from build123d import *

# Parameters (mm, degrees)
SKETCH_1_R      = 150
SKETCH_1_R_2    = 3
SKETCH_1_R_3    = 1.55
SKETCH_1_R_4    = 1
EXTRUDE_1_DEPTH = 3


with BuildPart() as part:
    # 草图1 → 凸台-拉伸1 (new body)
    with BuildSketch(Plane(origin=(0, 0, 0), x_dir=(1, 0, 0), z_dir=(0, 1, 0))):
        with Locations(Location((0, 0, 0), (0, 0, 270))):
            Circle(SKETCH_1_R)
        with Locations(Location((0, 0, 0), (0, 0, 270))):
            Circle(SKETCH_1_R_2, mode=Mode.SUBTRACT)
        with Locations(Location((0, 10, 0), (0, 0, 270))):
            Circle(SKETCH_1_R_3, mode=Mode.SUBTRACT)
        with Locations(Location((10, 0, 0), (0, 0, 270))):
            Circle(SKETCH_1_R_3, mode=Mode.SUBTRACT)
        with Locations(Location((0, -10, 0), (0, 0, 270))):
            Circle(SKETCH_1_R_3, mode=Mode.SUBTRACT)
        with Locations(Location((-10, 0, 0), (0, 0, 270))):
            Circle(SKETCH_1_R_3, mode=Mode.SUBTRACT)
        with Locations(Location((0, 125, 0), (0, 0, 270))):
            Circle(SKETCH_1_R_4, mode=Mode.SUBTRACT)
        with Locations(Location((17.67766953, 117.67766953, 0), (0, 0, 270))):
            Circle(SKETCH_1_R_4, mode=Mode.SUBTRACT)
        with Locations(Location((25, 100, 0), (0, 0, 270))):
            Circle(SKETCH_1_R_4, mode=Mode.SUBTRACT)
        with Locations(Location((17.67766953, 82.32233047, 0), (0, 0, 270))):
            Circle(SKETCH_1_R_4, mode=Mode.SUBTRACT)
        with Locations(Location((0, 75, 0), (0, 0, 270))):
            Circle(SKETCH_1_R_4, mode=Mode.SUBTRACT)
        with Locations(Location((-17.67766953, 82.32233047, 0), (0, 0, 270))):
            Circle(SKETCH_1_R_4, mode=Mode.SUBTRACT)
        with Locations(Location((-25, 100, 0), (0, 0, 270))):
            Circle(SKETCH_1_R_4, mode=Mode.SUBTRACT)
        with Locations(Location((-17.67766953, 117.67766953, 0), (0, 0, 270))):
            Circle(SKETCH_1_R_4, mode=Mode.SUBTRACT)
        with Locations(Location((0, 100, 0), (0, 0, 270))):
            Circle(SKETCH_1_R_4, mode=Mode.SUBTRACT)
        with Locations(Location((110.750686036, -43.529523872, 0), (0, 0, 270))):
            Circle(SKETCH_1_R_4, mode=Mode.SUBTRACT)
        with Locations(Location((108.253175473, -62.5, 0), (0, 0, 270))):
            Circle(SKETCH_1_R_4, mode=Mode.SUBTRACT)
        with Locations(Location((93.073016506, -74.148145657, 0), (0, 0, 270))):
            Circle(SKETCH_1_R_4, mode=Mode.SUBTRACT)
        with Locations(Location((99.102540378, -28.349364905, 0), (0, 0, 270))):
            Circle(SKETCH_1_R_4, mode=Mode.SUBTRACT)
        with Locations(Location((86.602540378, -50, 0), (0, 0, 270))):
            Circle(SKETCH_1_R_4, mode=Mode.SUBTRACT)
        with Locations(Location((80.132064251, -25.851854343, 0), (0, 0, 270))):
            Circle(SKETCH_1_R_4, mode=Mode.SUBTRACT)
        with Locations(Location((64.951905284, -37.5, 0), (0, 0, 270))):
            Circle(SKETCH_1_R_4, mode=Mode.SUBTRACT)
        with Locations(Location((62.454394721, -56.470476128, 0), (0, 0, 270))):
            Circle(SKETCH_1_R_4, mode=Mode.SUBTRACT)
        with Locations(Location((74.102540378, -71.650635095, 0), (0, 0, 270))):
            Circle(SKETCH_1_R_4, mode=Mode.SUBTRACT)
        with Locations(Location((-93.073016506, -74.148145657, 0), (0, 0, 270))):
            Circle(SKETCH_1_R_4, mode=Mode.SUBTRACT)
        with Locations(Location((-108.253175473, -62.5, 0), (0, 0, 270))):
            Circle(SKETCH_1_R_4, mode=Mode.SUBTRACT)
        with Locations(Location((-110.750686036, -43.529523872, 0), (0, 0, 270))):
            Circle(SKETCH_1_R_4, mode=Mode.SUBTRACT)
        with Locations(Location((-74.102540378, -71.650635095, 0), (0, 0, 270))):
            Circle(SKETCH_1_R_4, mode=Mode.SUBTRACT)
        with Locations(Location((-86.602540378, -50, 0), (0, 0, 270))):
            Circle(SKETCH_1_R_4, mode=Mode.SUBTRACT)
        with Locations(Location((-62.454394721, -56.470476128, 0), (0, 0, 270))):
            Circle(SKETCH_1_R_4, mode=Mode.SUBTRACT)
        with Locations(Location((-64.951905284, -37.5, 0), (0, 0, 270))):
            Circle(SKETCH_1_R_4, mode=Mode.SUBTRACT)
        with Locations(Location((-80.132064251, -25.851854343, 0), (0, 0, 270))):
            Circle(SKETCH_1_R_4, mode=Mode.SUBTRACT)
        with Locations(Location((-99.102540378, -28.349364905, 0), (0, 0, 270))):
            Circle(SKETCH_1_R_4, mode=Mode.SUBTRACT)
    extrude(amount=EXTRUDE_1_DEPTH)


solid = part.part
Geometry check sheet. Reference: the model listing, model coordinates, mm. Round coordinates to 2 decimals unless told otherwise and drop trailing zeros. Write each loop counter-clockwise with the first axis right and the second up, starting at its lowest first coordinate (ties: lowest second). Pieces come first, ordered by that corner, then holes.
Item 1: Material ranges on line 1 along X through (y, z) = (1.3, -100); line 2 along X through (y, z) = (0.9, -0.5); line 3 along X through (y, z) = (2.6, 49.5), recorded low to high.
Determined:
line 1: x = -111.8 to -26, -24 to -1, 1 to 24, 26 to 111.8
line 2: x = -150 to -11.47, -8.53 to -2.96, 2.96 to 8.53, 11.47 to 150
line 3: x = -141.6 to -87.47, -85.74 to 85.74, 87.47 to 141.6
Item 2: Section check C-C (z = -112). Record the boundary of the cut face in (x, y), plus the area to 3 significant figures.
Determined:
outline: (-99.78, 0) - (99.78, 0) - (99.78, 3) - (-99.78, 3) - close
area: 599 mm2
Item 3: Section check A-A (y = 2.15). Give the number of separate pieces and of enclosed holes in the cut face, plus the area to 3 significant figures.
Determined:
separate pieces: 1
enclosed holes: 32
area: 70,500 mm2
Item 4: Go/stop test with flat-tipped pins: pin 1 Ø1.5 at (x, y) = (77, 2) entering from -Z; pin 2 Ø1.5 at (y, z) = (2, 28) entering from -X. Record where each tip stops, or that it passes through.
Determined:
pin 1: stops at z = -129.17
pin 2: stops at x = -147.5
Item 5: Section check B-B (z = -30.5). Record the boundary of the cut face in (x, y).
Determined:
outline: (-146.87, 0) - (146.87, 0) - (146.87, 3) - (-146.87, 3) - close
